Model file for the job. Use its own axes, mm. A direction names the side the tool comes from. Coordinates: 2 decimals unless noted, no trailing zeros. Write each loop counter-clockwise with the first axis right and the second up, starting at its lowest first coordinate (ties: lowest second). Pieces come first, ordered by that corner, then holes. Notation, with made-up numbers: M 60,-33.5 L 80,-33.5 A33 cw 80,0.5 Z; hole C 64.5,-4.5 d8. An arc over 180 degrees is marked long. Use CSV: the item, a comma, the result in double quotes. Start each with the question number.
from build123d import *

# Parameters (mm, degrees)
SKETCH1_W           = 50
SKETCH1_H           = 160
BOSS_EXTRUDE1_DEPTH = 3
FILLET2_R           = 15
CUT_EXTRUDE1_DEPTH  = 4


with BuildPart() as part:
    # Sketch1 → Boss-Extrude1 (new body)
    with BuildSketch(Plane(origin=(0, 0, 0), x_dir=(1, 0, 0), z_dir=(0, 1, 0))):
        Rectangle(SKETCH1_W, SKETCH1_H)
    extrude(amount=BOSS_EXTRUDE1_DEPTH)

    # Fillet2
    fillet2_edges = [part.edges().sort_by_distance(p)[0] for p in [
        (25, 1.5, 80),
        (-25, 1.5, 80),
        (-25, 1.5, -80),
        (25, 1.5, -80),
    ]]
    fillet(fillet2_edges, radius=FILLET2_R)

    # Sketch3 → Cut-Extrude1 (cut, through all)
    with BuildSketch(Plane(origin=(0, 3, 0), x_dir=(1, 0, 0), z_dir=(0, 1, 0))):
        with BuildLine():
            Line((-12.1, 70), (12.1, 70))
            ThreePointArc((12.1, 70), (14.221320344, 69.121320344), (15.1, 67))
            Line((15.1, 67), (15.1, 12.8))
            ThreePointArc((15.1, 12.8), (14.221320344, 10.678679656), (12.1, 9.8))
            Line((12.1, 9.8), (-12.1, 9.8))
            ThreePointArc((-12.1, 9.8), (-14.221320344, 10.678679656), (-15.1, 12.8))
            Line((-15.1, 12.8), (-15.1, 67))
            ThreePointArc((-15.1, 67), (-14.221320344, 69.121320344), (-12.1, 70))
        make_face()
    cut_extrude1 = extrude(amount=-CUT_EXTRUDE1_DEPTH, mode=Mode.SUBTRACT)

    # Mirror1: Cut-Extrude1 across plane
    add(cut_extrude1.mirror(Plane.XY), mode=Mode.SUBTRACT)


solid = part.part
1) Drop a flat-ended pin along its axis: P1, Ø1.5, axis at x = -12, y = 2, coming from the -Z side. Give the stop position or say it passes through.
2) Wall check: L1, parallel to Z at x = 7, y = 0.8; L2, parallel to X at y = 0.3, z = -57; L3, parallel to Z at x = -12.5, y = 1.85. Give the ranges that are in metal, low to high. Write a range as [from, to].
3) Tool access for faces 1 (the face through (-20.72, 1.52, -75.49)), 2 (the face through (14.24, 1.52, 10.7)): list every direction of +Z, -Z, +X, -X, +Y, -Y with a clear straight run to the whole face (end or side of a thin tool).
4) Band-saw the part on D-D on x = 21.5. List the corners of the cut face in (y, z), then the cut area to 3 significant figures.
5) Band-saw the part on C-C on x = 8. List the corners of the cut face in (y, z).
6) Two-plate mould, pull along X, no slides. Class faces 3 (the face through (0, 1, 80)), 4 (the face through (15.1, 2, -40)), 5 (the face through (-20.72, 1.52, 75.49)): pulls with the +X half, pulls with the -X half, needs draft (parallel to the pull), parting line crosses it, or undercut.
7) Band-saw the part on B-B on z = -32. List the corners of the cut face in (x, y).
8) Band-saw the part on A-A on y = 0.55. List the corners of the cut face in (x, z), then the cut area to 3 significant figures.
Findings below:
1,P1,"stops at z = -79.95"
2,L1,"z = [-80, -70], [-9.8, 9.8], [70, 80]"
2,L2,"x = [-25, -15.1], [15.1, 25]"
2,L3,"z = [-79.79, -69.97], [-9.83, 9.83], [69.97, 79.79]"
3,face 1,"-Z, -X, +Y, -Y"
3,face 2,"+Y, -Y"
4,outline,"M 0,-74.63 L 3,-74.63 L 3,74.63 L 0,74.63 Z"
4,area,"448 mm2"
5,outline,"M 0,-80 L 3,-80 L 3,-70 L 0,-70 Z; M 0,-9.8 L 3,-9.8 L 3,9.8 L 0,9.8 Z; M 0,70 L 3,70 L 3,80 L 0,80 Z"
6,face 3,"needs draft"
6,face 4,"undercut"
6,face 5,"pulls with the -X half"
7,outline,"M -25,0 L -15.1,0 L -15.1,3 L -25,3 Z; M 15.1,0 L 25,0 L 25,3 L 15.1,3 Z"
8,outline,"M -25,-65 A15 ccw -10,-80 L 10,-80 A15 ccw 25,-65 L 25,65 A15 ccw 10,80 L -10,80 A15 ccw -25,65 Z; hole M -15.1,-67 A3 ccw -12.1,-70 L 12.1,-70 A3 ccw 15.1,-67 L 15.1,-12.8 A3 ccw 12.1,-9.8 L -12.1,-9.8 A3 ccw -15.1,-12.8 Z; hole M -15.1,12.8 A3 ccw -12.1,9.8 L 12.1,9.8 A3 ccw 15.1,12.8 L 15.1,67 A3 ccw 12.1,70 L -12.1,70 A3 ccw -15.1,67 Z"
8,area,"4,190 mm2"
